The drawing under review shows one solid part. Ordinate dimensions are in mm from its lowest x, y, z. Coordinates: 2 decimals unless noted, no trailing zeros. Write each loop counter-clockwise with the first axis right and the second up, starting at its lowest first coordinate (ties: lowest second). Pieces come first, ordered by that corner, then holes. Notation, with made-up numbers: M -11.5,-4.75 L 22.5,-4.75 A22 cw 22.5,32.25 Z; hole C 65.25,-10 d2. An arc over 180 degrees is marked long. Write item = value, one per line.
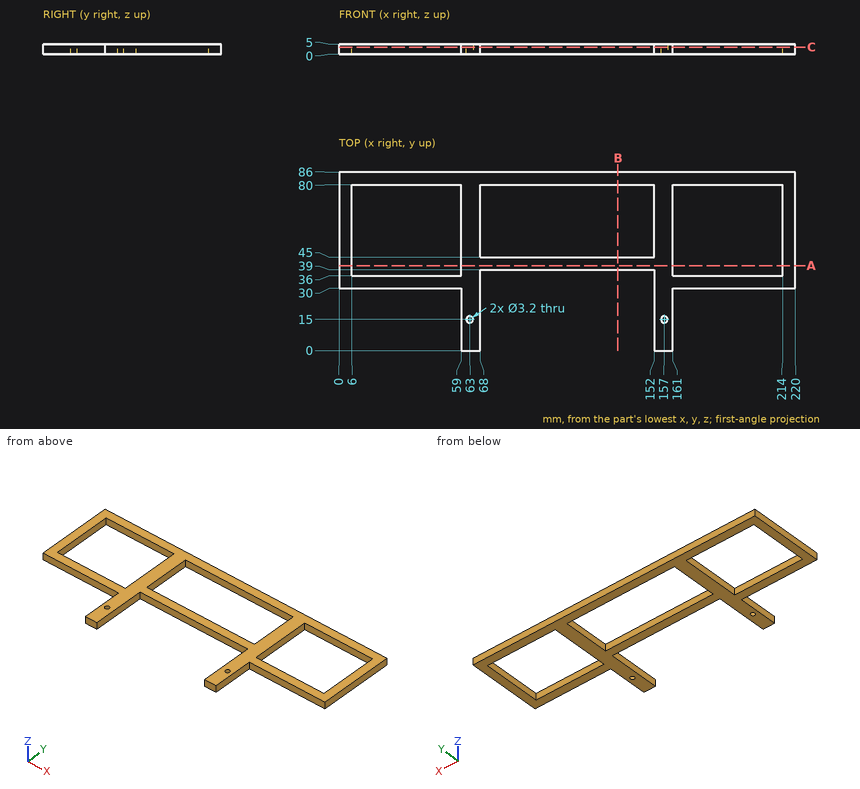
Q1. Consider section B-B, the plane x = 134.5. State the section outline as (y, z) points, and give its area (3 significant figures).
Check result:
outline = M 39,0 L 45,0 L 45,5 L 39,5 Z; M 80,0 L 86,0 L 86,5 L 80,5 Z
area = 60.0 mm²
Q2. Consider section C-C, the plane z = 3.5. State the section outline as (x, y) points.
Check result:
outline = M 0,30 L 59,30 L 59,0 L 68,0 L 68,39 L 152,39 L 152,0 L 161,0 L 161,30 L 220,30 L 220,86 L 0,86 Z; hole M 6,36 L 59,36 L 59,80 L 6,80 Z; hole C 63,15 d3.2; hole M 68,45 L 152,45 L 152,80 L 68,80 Z; hole C 157,15 d3.2; hole M 161,36 L 214,36 L 214,80 L 161,80 Z
Q3. Consider section A-A, the plane y = 41. State the section outline as (x, z) points.
Check result:
outline = M 0,0 L 6,0 L 6,5 L 0,5 Z; M 59,0 L 161,0 L 161,5 L 59,5 Z; M 214,0 L 220,0 L 220,5 L 214,5 Z
Q4. Wall thickness on line 1 (X direction, y = 46, z = 1.5); line 2 (X direction, y = 44.5, z = 4.1); line 3 (Y direction, x = 157, z = 3.9): over which ranges is each line inside the solid? List them lowest first.
Check result:
line_1 = 0 to 6, 59 to 68, 152 to 161, 214 to 220
line_2 = 0 to 6, 59 to 161, 214 to 220
line_3 = 0 to 13.4, 16.6 to 86
Q5. For P1, Ø1.5, axis at x = 108, z = 2.5, coming from the -Y side; P2, Ø1.5, axis at y = 28, z = 3, coming from the -X side; P3, Ø3, axis at x = 175, z = 2, coming from the -Y side, all flat-tipped, find the tip position at first contact; note any pin that passes through.
Check result:
P1 = 39
P2 = 59
P3 = 30
